Could you check a few things on this model? Use its own coordinates, in mm. Give positions to 0.01 mm unless a question says otherwise; leave off trailing zeros. Order: outer loops, then holes, each group sorted by start corner. A loop starts at its lowest first (then second) coordinate and runs counter-clockwise, first axis right, second up. Notation, with made-up numbers: (-5.75, -4.5) - (16.25, -4.5) arc R12 cw to (16.25, 15.5) - close; hole circle Ø5 at (57, 4). An arc over 180 degrees is marked (long way). One line per question, with ' | ' between items. Start each with the question number.
1. I need wall thicknesses on probe 1 along X at (y, z) = (-24, 1.65); probe 2 along Y at (x, z) = (-33, 1.15). Which ranges of each line are inside material? Lowest first, please. Write a range as from..to.
2. For P1, Ø1.5, axis at y = -25, z = 2.5, coming from the +X side; P2, Ø2.5, axis at x = -103, z = 2.5, coming from the +Y side; P3, Ø2.5, axis at x = -39.5, z = 2.5, coming from the -Y side; P4, Ø3, axis at y = -23.5, z = 4.5, coming from the -X side, each with a flat end and sliding along its axis, tell me the tip position at first contact or that it passes through.
3. Imagine slicing it at B-B (x = -43.5). Please give me the cut outline in (y, z), and give its area (3 significant figures).
4. Imagine slicing it at A-A (z = 4.2). Please give me the cut outline in (x, y), and give its area (3 significant figures).
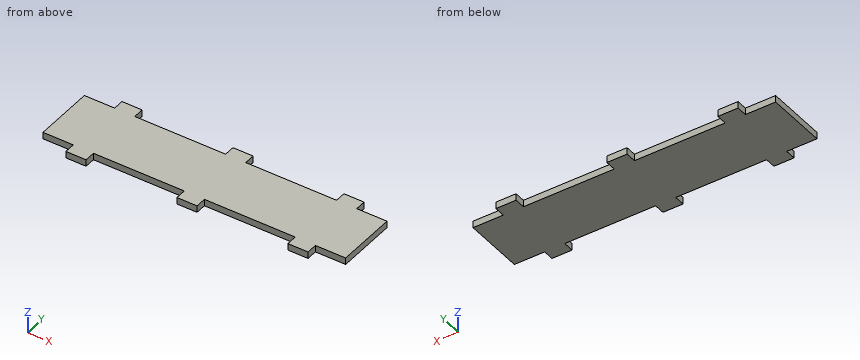
```python
from build123d import *

# Parameters (mm, degrees)
F1_DEPTH = 5


with BuildPart() as f1:
    # F0 (on Top) → F1 (new body)
    with BuildSketch(Plane.XY):
        Polygon((112.5, 0), (-112.5, 0), (-112.5, -22.5), (-90, -22.5), (-90, -30.5), (-75, -30.5), (-75, -22.5), (-7.5, -22.5), (-7.5, -30.5), (7.5, -30.5), (7.5, -22.5), (75, -22.5), (75, -30.5), (90, -30.5), (90, -22.5), (112.5, -22.5), align=None)
        Polygon((-112.5, 22.5), (-112.5, 0), (112.5, 0), (112.5, 22.5), (90, 22.5), (90, 30.5), (75, 30.5), (75, 22.5), (7.5, 22.5), (7.5, 30.5), (-7.5, 30.5), (-7.5, 22.5), (-75, 22.5), (-75, 30.5), (-90, 30.5), (-90, 22.5), align=None)
    extrude(amount=F1_DEPTH)


solid = f1.part
```
Results found:
1) probe 1: x = -90..-75, -7.5..7.5, 75..90 | probe 2: y = -22.5..22.5
2) P1: stops at x = 90 | P2: stops at y = 22.5 | P3: stops at y = -22.5 | P4: stops at x = -112.5
3) outline: (-22.5, 0) - (22.5, 0) - (22.5, 5) - (-22.5, 5) - close | area: 225 mm2
4) outline: (-112.5, -22.5) - (-90, -22.5) - (-90, -30.5) - (-75, -30.5) - (-75, -22.5) - (-7.5, -22.5) - (-7.5, -30.5) - (7.5, -30.5) - (7.5, -22.5) - (75, -22.5) - (75, -30.5) - (90, -30.5) - (90, -22.5) - (112.5, -22.5) - (112.5, 22.5) - (90, 22.5) - (90, 30.5) - (75, 30.5) - (75, 22.5) - (7.5, 22.5) - (7.5, 30.5) - (-7.5, 30.5) - (-7.5, 22.5) - (-75, 22.5) - (-75, 30.5) - (-90, 30.5) - (-90, 22.5) - (-112.5, 22.5) - close | area: 10,800 mm2
